from build123d import *

# Parameters (mm, degrees)
SKETCH2_R               = 20
SKETCH2_R_2             = 3
BOSS_EXTRUDE1_DEPTH     = 3
BOSS_EXTRUDE2_START     = 3
SKETCH5_R               = 1.5
BOSS_EXTRUDE2_DEPTH     = 7
CUT_EXTRUDE1_DEPTH      = 8
CUT_EXTRUDE1_DEPTH_BACK = 8
SKETCH6_R               = 0.300327284
BOSS_EXTRUDE3_DEPTH     = 3
SKETCH8_R               = 2.130430509
BOSS_EXTRUDE4_DEPTH     = 2


with BuildPart() as part:
    # Sketch2 → Boss-Extrude1 (new body)
    with BuildSketch(Plane(origin=(0, 0, 0), x_dir=(1, 0, 0), z_dir=(0, 1, 0))):
        with Locations(Location((0, 0, 0), (0, 0, 270))):
            Circle(SKETCH2_R)
        with Locations(Location((0, 0, 0), (0, 0, 270))):
            Circle(SKETCH2_R_2, mode=Mode.SUBTRACT)
    extrude(amount=BOSS_EXTRUDE1_DEPTH)

    # Sketch5 → Boss-Extrude2 (add)
    with BuildSketch(Plane(origin=(0, 0, 0), x_dir=(1, 0, 0), z_dir=(0, 1, 0)).offset(BOSS_EXTRUDE2_START)):
        with Locations(Location((17.949264284, 0, 0), (0, 0, 270))):
            Circle(SKETCH5_R)
    extrude(amount=BOSS_EXTRUDE2_DEPTH)

    # Sketch6 → Cut-Extrude1 (cut, two sides: drawn at the far end of the back side and taken through both)
    with BuildSketch(Plane.XY.offset(-CUT_EXTRUDE1_DEPTH_BACK)):
        with Locations(Location((17.939875417, 8.605457477, 0), (0, 0, 180))):
            Circle(SKETCH6_R)
    extrude(amount=CUT_EXTRUDE1_DEPTH + CUT_EXTRUDE1_DEPTH_BACK, mode=Mode.SUBTRACT)

    # Sketch7 → Boss-Extrude3 (add)
    with BuildSketch(Plane(origin=(0, 0, 0), x_dir=(1, 0, 0), z_dir=(0, 1, 0))):
        with BuildLine():
            Line((-3, 0), (0, 3))
            ThreePointArc((0, 3), (-2.121320344, 2.121320344), (-3, 0))
        make_face()
    extrude(amount=BOSS_EXTRUDE3_DEPTH)

    # Sketch8 → Boss-Extrude4 (add)
    with BuildSketch(Plane(origin=(0, 3, 0), x_dir=(1, 0, 0), z_dir=(0, 1, 0))):
        with Locations(Location((17.949264284, 0, 0), (0, 0, 16.617512863))):
            Circle(SKETCH8_R)
    extrude(amount=BOSS_EXTRUDE4_DEPTH)


solid = part.part
The model under review builds one solid part; all positions refer to its coordinate system, in mm. A direction names the side the tool comes from. Round coordinates to 2 decimals unless told otherwise and drop trailing zeros. Loops run counter-clockwise (first coordinate to the right, second up) from the corner with the lowest first, then second, coordinate; pieces in that order, holes last. Notation, with made-up numbers: (-7, -32.5) -> (-3, -32.5) arc R20 cw to (-3, -9.5) -> close; hole circle Ø11 at (63.5, -32.5). An arc over 180 degrees is marked (long way). Return JSON: item names as keys, results as strings.
(1) The part is to be moulded in two halves that separate along Z. For faces 1 (the flat face through (0, 0, 4)), 2 (the cylindrical face through (2.05, 1.48, 2.19)), 3 (the flat face through (-2, 1, -1)), 4 (the cylindrical face through (16.033, 3.986, -0.931)), say which applies: released by +Z, released by -Z, zero draft, split by the parting line, or undercut.
Solved:
{"face 1": "zero draft", "face 2": "undercut", "face 3": "undercut", "face 4": "split by the parting line"}
(2) Add section B-B on x = -1.5. Write out the cut boundary in (y, z).
Solved:
{"outline": "(0, -19.94) -> (3, -19.94) -> (3, -1.5) -> (0, -1.5) -> close; (0, 2.6) -> (3, 2.6) -> (3, 19.94) -> (0, 19.94) -> close"}
(3) Add section D-D on y = 3.75. Write out the cut boundary in (x, z), plus the area to 3 significant figures.
Solved:
{"outline": "circle Ø4.26 at (17.95, 0)", "area": "14.3 mm2"}
(4) For line 1 (Z direction, x = 0, y = 1.75); line 2 (Y direction, x = 17, z = 9.5), list the stretches that pass through material, from the lowest coordinate up.
Solved:
{"line 1": "-20 to -3, 3 to 20", "line 2": "0 to 3"}
(5) For faces 5 (the flat face through (16, 5, 0)), 6 (the flat face through (18, 10, 0)), list the 3-axis set-ups (+Z, -Z, +X, -X, +Y, -Y) from which the entire face can be reached by the end or side of a thin tool; tool diameter is ignored.
Solved:
{"face 5": "+Y", "face 6": "+Z, -Z, +X, -X, +Y"}
(6) Add section C-C on x = 17. Write out the cut boundary in (y, z), plus the area to 3 significant figures.
Solved:
{"outline": "(0, -10.54) -> (3, -10.54) -> (3, -1.91) -> (5, -1.91) -> (5, -1.16) -> (10, -1.16) -> (10, 1.16) -> (5, 1.16) -> (5, 1.91) -> (3, 1.91) -> (3, 10.54) -> (0, 10.54) -> close", "area": "82.5 mm2"}
(7) For pin 1 (7 mm diameter, centred on x = 0, z = 0, fed in from +Y); pin 2 (6 mm diameter, centred on y = 5.5, z = 9.5, fed in from +X), all flat-tipped, find the tip position at first contact; note any pin that passes through.
Solved:
{"pin 1": "y = 3", "pin 2": "x = 18.4"}
(8) Add section A-A on y = 1.25. Write out the cut boundary in (x, z).
Solved:
{"outline": "circle Ø40 at (0, 0); hole (-3, 0) -> (0, -3) arc R3 ccw (long way) to start"}
